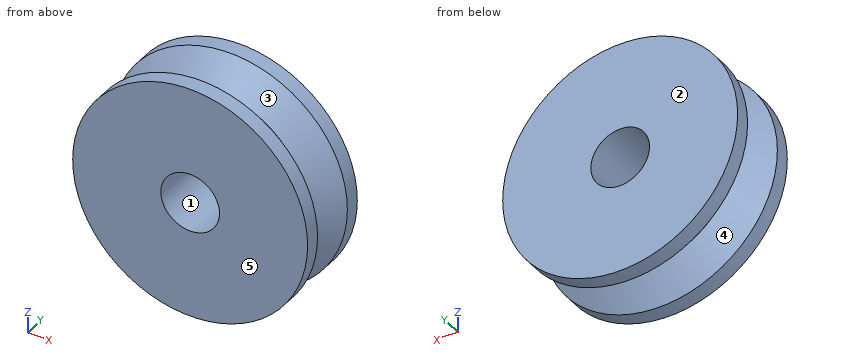
```python
from build123d import *

# Parameters (mm, degrees)
SKETCH1_R           = 6
SKETCH1_R_2         = 1.5
BOSS_EXTRUDE1_DEPTH = 4


with BuildPart() as part:
    # Sketch1 → Boss-Extrude1 (new body)
    with BuildSketch(Plane(origin=(0, 0, 0), x_dir=(1, 0, 0), z_dir=(0, 1, 0))):
        Circle(SKETCH1_R)
        Circle(SKETCH1_R_2, mode=Mode.SUBTRACT)
    extrude(amount=BOSS_EXTRUDE1_DEPTH)

    # Cut-Sweep3: sweep along a path in Sketch3
    with BuildLine(Plane(origin=(0, 2, 0), x_dir=(1, 0, 0), z_dir=(0, 1, 0))) as cut_sweep3_path:
        CenterArc((0, 0), 6, 0, 360)
    # Sketch2 → Cut-Sweep3 (sweep, cut)
    with BuildSketch(Plane.XY):
        Polygon((-6, 3.2), (-6, 0.8), (-4.75, 2), align=None)
    sweep(path=cut_sweep3_path.line, mode=Mode.SUBTRACT)


solid = part.part
```
Part model, mm, in its own coordinate system. Face numbers are marked on the shaded views. A direction names the side the tool comes from. Coordinates: 2 decimals unless noted, no trailing zeros. Write each loop counter-clockwise with the first axis right and the second up, starting at its lowest first coordinate (ties: lowest second). Pieces come first, ordered by that corner, then holes.
Item 1: Mould opens along Y. For the marked faces 1, 2 and 3 say: released by +Y, released by -Y, zero draft, split by the parting line, or undercut.
Item 2: Slice it at D-D (y = 2.15). Write the cut outline in (x, z).
Item 3: Which spindle directions (+Z, -Z, +X, -X, +Y, -Y) get a long thin tool onto all of the face, cutting with end or side? Do the marked faces 4 and 5. Say none if no direction does.
Item 4: Slice it at C-C (y = 1). Write the cut outline in (x, z), and give its area (3 significant figures).
Item 5: Probe line 1 (Z direction, x = 0, y = 2.5); line 2 (Z direction, x = -0.5, y = 1.35); line 3 (X direction, y = 3, z = -0.5). List the from-to ranges inside material, lowest first.
Item 6: Slice it at B-B (z = 0). Write the cut outline in (x, y).
Item 7: Slice it at A-A (x = 0). Write the cut outline in (y, z).
Item 8: Pin check, flat tip, straight feed: pin 1 (1 mm diameter, centred on y = 1.5, z = 4, fed in from -X). Stop position of the tip, or through.
Results found:
1. face 1: zero draft
1. face 2: released by +Y
1. face 3: undercut
2. outline: circle Ø9.81 at (0, 0); hole circle Ø3 at (0, 0)
3. face 4: none
3. face 5: +Z, -Z, +X, -X, -Y
4. outline: circle Ø11.58 at (0, 0); hole circle Ø3 at (0, 0)
4. area: 98.3 mm2
5. line 1: z = -5.27 to -1.5, 1.5 to 5.27
5. line 2: z = -5.4 to -1.41, 1.41 to 5.4
5. line 3: x = -5.77 to -1.41, 1.41 to 5.77
6. outline: (-6, 0) - (-1.5, 0) - (-1.5, 4) - (-6, 4) - (-6, 3.2) - (-4.75, 2) - (-6, 0.8) - close; (1.5, 0) - (6, 0) - (6, 0.8) - (4.75, 2) - (6, 3.2) - (6, 4) - (1.5, 4) - close
7. outline: (0, -6) - (0.8, -6) - (2, -4.75) - (3.2, -6) - (4, -6) - (4, -1.5) - (0, -1.5) - close; (0, 1.5) - (4, 1.5) - (4, 6) - (3.2, 6) - (2, 4.75) - (0.8, 6) - (0, 6) - close
8. pin 1: stops at x = -4.32
